from build123d import *

# Parameters (mm, degrees)
SKETCH1_W          = 498.475
SKETCH1_H          = 355.6
BASE_FLANGE1_DEPTH = 1.1938
CUT_EXTRUDE1_REACH = 308.159
SKETCH6_R          = 4.7625
FILLET1_R          = 6.35


# Sheet-metal steps are written as plain solids
with BuildPart() as part:
    # Sketch1 → Base-Flange1 (new body)
    with BuildSketch(Plane(origin=(0, 0, 0), x_dir=(0, 0, -1), z_dir=(1, 0, 0))):
        Rectangle(SKETCH1_W, SKETCH1_H)
    extrude(amount=-BASE_FLANGE1_DEPTH)

    # Sketch6 → Cut-Extrude1 (cut, up to next)
    with BuildSketch(Plane(origin=(0, 0, 0), x_dir=(0, 0, -1), z_dir=(1, 0, 0)), mode=Mode.PRIVATE) as cut_extrude1_sk1:
        with Locations((-152.4, 163.5125)):
            Circle(SKETCH6_R)
    cut_extrude1_tool1 = extrude(cut_extrude1_sk1.sketch, amount=-CUT_EXTRUDE1_REACH, mode=Mode.PRIVATE) & part.part
    # Sketch6 → Cut-Extrude1 (cut, up to next)
    with BuildSketch(Plane(origin=(0, 0, 0), x_dir=(0, 0, -1), z_dir=(1, 0, 0)), mode=Mode.PRIVATE) as cut_extrude1_sk2:
        with Locations((-234.95, 0)):
            Circle(SKETCH6_R)
    cut_extrude1_tool2 = extrude(cut_extrude1_sk2.sketch, amount=-CUT_EXTRUDE1_REACH, mode=Mode.PRIVATE) & part.part
    cut_extrude1_1 = cut_extrude1_tool1.solids().sort_by_distance((0, 163.5125, 152.4))[0]
    add(cut_extrude1_1, mode=Mode.SUBTRACT)
    cut_extrude1_2 = cut_extrude1_tool2.solids().sort_by_distance((0, 0, 234.95))[0]
    add(cut_extrude1_2, mode=Mode.SUBTRACT)
    cut_extrude1 = cut_extrude1_1 + cut_extrude1_2  # Cut-Extrude1 as one shape, for the pattern or mirror that repeats it

    # Mirror1: Cut-Extrude1 across plane
    add(cut_extrude1.mirror(Plane.XY), mode=Mode.SUBTRACT)

    # Fillet1
    fillet1_edges = [part.edges().sort_by_distance(p)[0] for p in [
        (-0.5969, 177.8, 249.2375),
        (-0.5969, 177.8, -249.2375),
        (-0.5969, -177.8, -249.2375),
        (-0.5969, -177.8, 249.2375),
    ]]
    fillet(fillet1_edges, radius=FILLET1_R)


solid = part.part
Build history of the part. All positions in model axes, mm. Give positions to 0.01 mm unless a question says otherwise; leave off trailing zeros. Put each result on its own line as item: value.
Item 1: Two-plate mould, pull along Z, no slides. Class faces 1 (the cylindrical face through (-0.6, 1.4, 230.4)), 2 (the flat face through (0, 2, 3)): +Z half, -Z half, draft (parallel to the pull), parting line (faces both ways), or undercut.
From the geometry:
face 1: undercut
face 2: draft
Item 2: Probe line 1 (Y direction, x = -0.9, z = 234.95); line 2 (Y direction, x = -0.35, z = 152.4) (3 decimals); line 3 (Z direction, x = -0.55, y = -3). List the from-to ranges inside material, lowest first. Write a range as [from, to].
From the geometry:
line 1: y = [-177.8, -4.76], [4.76, 177.8]
line 2: y = [-177.8, 158.75], [168.275, 177.8]
line 3: z = [-249.24, -238.65], [-231.25, 231.25], [238.65, 249.24]
Item 3: Flat gauge pin, fed straight in: pin 1 Ø7.5 at (y, z) = (0, -234.95) entering from -X. Where does the tip first touch, or does it go through?
From the geometry:
pin 1: passes through
